Geometry: see drawing. Coordinates: mm, zero at the bounding-box minimum. Give positions to 0.01 mm unless a question says otherwise; leave off trailing zeros. Write each loop counter-clockwise with the first axis right and the second up, starting at its lowest first coordinate (ties: lowest second). Pieces come first, ordered by that corner, then holes. Notation, with made-up numbers: (0, -6.75) -> (30, -6.75) arc R15 cw to (30, 0.25) -> close; hole circle Ø3 at (35.25, 35). An arc over 180 degrees is marked (long way). Answer as a JSON object with one key per item and string values. Group by question number.
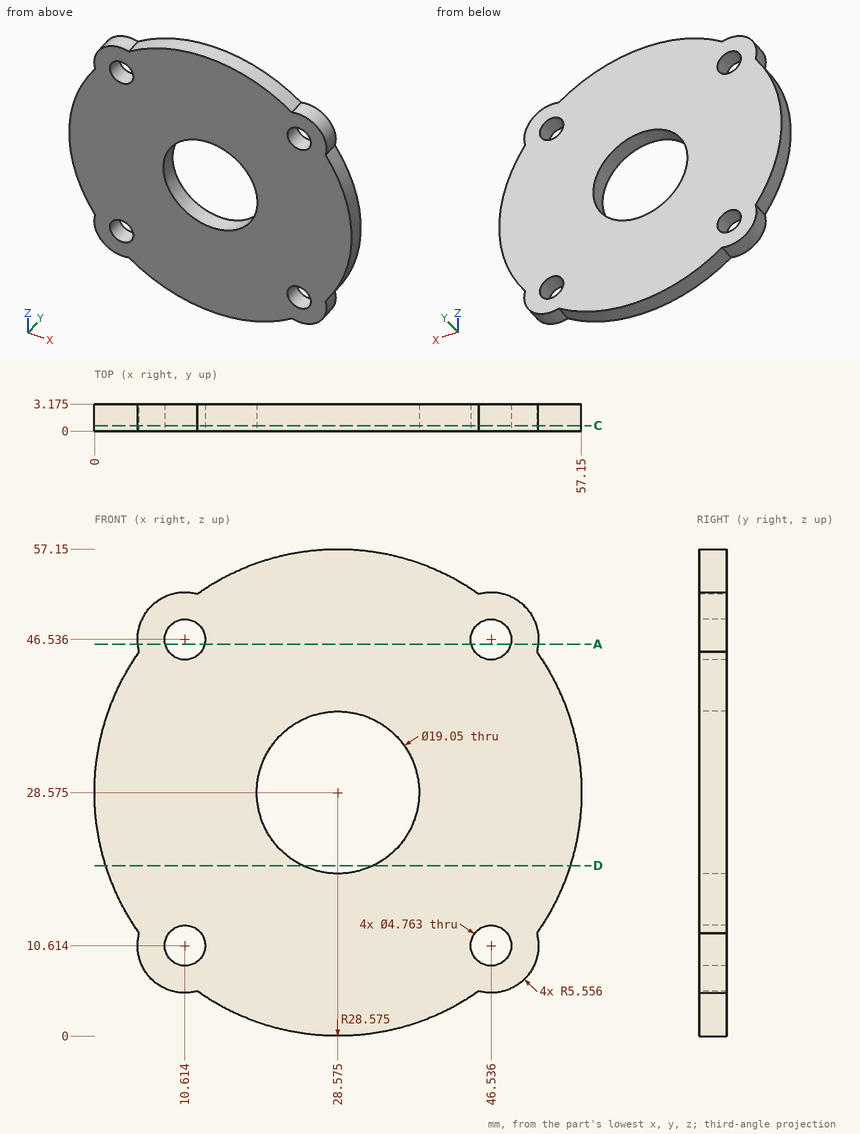
1. Line query: line 1 (X direction, y = 1.35, z = 8.5) (1 decimal); line 2 (X direction, y = 1.8, z = 35) (1 decimal); line 3 (X direction, y = 1.5, z = 29.5) (1 decimal). Output: solid intervals per line, ascending.
2. Section D-D (z = 20). Return the cut outline in (x, y) (1 decimal), plus the area to 3 significant figures.
3. Section C-C (y = 0.65). State how many separate pieces and enclosed holes the cut face has.
4. Section A-A (z = 46). Return the cut outline in (x, y) (1 decimal).
5. Contact query for flat-ended pins moving along their axis: pin 1 Ø1.5 at (x, y) = (14, 1.5) entering from +Z; pin 2 Ø3 at (x, z) = (46.54, 10.61) entering from +Y. Output: stop coordinate, or through.
Working result:
{
 "1": {"line 1": "x = 5.5 to 9.5, 11.7 to 45.4, 47.6 to 51.7", "line 2": "x = 0.7 to 21.5, 35.6 to 56.4", "line 3": "x = 0 to 19.1, 38.1 to 57.1"},
 "2": {"outline": "(1.3, 0) -> (24.4, 0) -> (24.4, 3.2) -> (1.3, 3.2) -> close; (32.7, 0) -> (55.8, 0) -> (55.8, 3.2) -> (32.7, 3.2) -> close", "area": "147 mm^2"},
 "3": {"separate pieces": "1", "enclosed holes": "5"},
 "4": {"outline": "(5.1, 0) -> (8.3, 0) -> (8.3, 3.2) -> (5.1, 3.2) -> close; (12.9, 0) -> (44.2, 0) -> (44.2, 3.2) -> (12.9, 3.2) -> close; (48.9, 0) -> (52.1, 0) -> (52.1, 3.2) -> (48.9, 3.2) -> close"},
 "5": {"pin 1": "stops at z = 53.58", "pin 2": "passes through"}
}
